Check sheet for the modelled part. Datum: model origin and axes. Units: mm. Coordinates: 2 decimals unless noted, no trailing zeros. Loops run counter-clockwise (first coordinate to the right, second up) from the corner with the lowest first, then second, coordinate; pieces in that order, holes last.
```python
from build123d import *

# Parameters (mm, degrees)
SALIENTE_EXTRUIR1_DEPTH = 2
CROQUIS2_R              = 6
CORTAR_EXTRUIR1_DEPTH   = 173.420996401


with BuildPart() as part:
    # Croquis1 → Saliente-Extruir1 (new body)
    with BuildSketch(Plane.XY):
        with BuildLine():
            Line((-150, 0), (-150, 85))
            Line((-150, 85), (150, 85))
            Line((150, 85), (150, 0))
            ThreePointArc((150, 0), (0, 35), (-150, 0))
        make_face()
    extrude(amount=SALIENTE_EXTRUIR1_DEPTH)

    # Croquis2 → Cortar-Extruir1 (cut, through all)
    with BuildSketch(Plane.XY.offset(2)):
        with Locations((-77, 72)):
            Circle(CROQUIS2_R)
        with Locations((77, 72)):
            Circle(CROQUIS2_R)
    extrude(amount=-CORTAR_EXTRUIR1_DEPTH, mode=Mode.SUBTRACT)


solid = part.part
```
1) Section check C-C on x = -77. Enter the section's corners in (y, z).
Answer sheet:
outline: (26.14, 0) - (66, 0) - (66, 2) - (26.14, 2) - close; (78, 0) - (85, 0) - (85, 2) - (78, 2) - close
2) Scan lines: line 1 (X direction, y = 75, z = 0.9); line 2 (Y direction, x = 77, z = 0.4); line 3 (X direction, y = 76, z = 1.2). Record each from-to range of solid material in increasing order.
Answer sheet:
line 1: x = -150 to -82.2, -71.8 to 71.8, 82.2 to 150
line 2: y = 26.14 to 66, 78 to 85
line 3: x = -150 to -81.47, -72.53 to 72.53, 81.47 to 150
3) Section check A-A on y = 72. Enter the section's corners in (x, z), plus the area to 3 significant figures.
Answer sheet:
outline: (-150, 0) - (-83, 0) - (-83, 2) - (-150, 2) - close; (-71, 0) - (71, 0) - (71, 2) - (-71, 2) - close; (83, 0) - (150, 0) - (150, 2) - (83, 2) - close
area: 552 mm2
4) Section check D-D on z = 1.7. Enter the section's corners in (x, y), plus the area to 3 significant figures.
Answer sheet:
outline: (-150, 0) arc R338.93 cw to (150, 0) - (150, 85) - (-150, 85) - close; hole circle Ø12 at (-77, 72); hole circle Ø12 at (77, 72)
area: 18,200 mm2
5) Mould release check, pull along Y, two halves, no side actions. Record for faces 1 (the cylindrical face through (2.175, 34.993, 0.986)), 2 (the flat face through (2, 53, 2)), 3 (the cylindrical face through (72.58, 76.06, 1.01)): +Y half, -Y half, draft (parallel to the pull), parting line (faces both ways), or undercut.
Answer sheet:
face 1: -Y half
face 2: draft
face 3: undercut
